Geometry check sheet. Reference: the model listing, model coordinates, mm. A direction names the side the tool comes from. Coordinates: 2 decimals unless noted, no trailing zeros. Write each loop counter-clockwise with the first axis right and the second up, starting at its lowest first coordinate (ties: lowest second). Pieces come first, ordered by that corner, then holes. Notation, with made-up numbers: M 65,12.25 L 72,12.25 A12 ccw 72,33.25 Z; hole C 30.5,-33.5 d3. An arc over 180 degrees is marked long. Put each result on its own line as item: value. Start each with the question number.
1) Cross-section at D-D on z = 43. Record the cut outline in (x, y), plus the area to 3 significant figures.
2) Scan lines: line 1 along Y through (x, z) = (0, 54); line 2 along X through (y, z) = (-25, 57); line 3 along X through (y, z) = (-41.5, 31). Record each from-to range of solid material in increasing order.
3) Set-up check for faces 5 (the flat face through (-5, 48.368, 75)), 6 (the cylindrical face through (-65.992, -68.182, 15.027)): record each of +Z, -Z, +X, -X, +Y, -Y from which the full face is reachable in a straight line by a thin tool's end or side.
4) Cross-section at A-A on x = 0. Record the cut outline in (y, z), plus the area to 3 significant figures.
5) Gauge pin test, flat ends, axial feed: pin 1 (10 mm diameter, centred on x = -87.5, y = -66, fed in from -Z); pin 2 (10 mm diameter, centred on y = -50, z = 106, fed in from -X). Record the tip position at first contact, or that the pin passes through.
6) Cross-section at B-B on y = 8. Record the cut outline in (x, z).
7) Mould release check, pull along X, two halves, no side actions. Record for faces 1 (the flat face through (-101, -69, 30.48)), 2 (the flat face through (-101, -58.402, 15)), 3 (the flat face through (-155.258, -29, 38)), 4 (the flat face through (149.542, -29, 75)): released by +X, released by -X, zero draft, split by the parting line, or undercut.
8) Cross-section at C-C on z = 25.5. Record the cut outline in (x, y), plus the area to 3 significant figures.
from build123d import *

# Parameters (mm, degrees)
F0_W     = 304.8
F0_H     = 152.4
F1_DEPTH = 152.4
F9_R     = 30.48
F5_DEPTH = 152.401
F6_SIZE  = 76.2
F8_DEPTH = 30.48


# Not quite as in the source:
# - the program builds the solid bodies; features that only make, move or delete a surface that nothing else refers to are left out


with BuildPart() as f1:
    # F0 (on Top) → F1 (new body)
    with BuildSketch(Plane.XY):
        with Locations((-2.8575006872, -27.8319329938)):
            Rectangle(F0_W, F0_H)
    extrude(amount=F1_DEPTH)

    # F9 (on face) → F5 (cut, through all)
    with BuildSketch(Plane.XY.offset(152.4)):
        with Locations((0, -15.3043069538)):
            Circle(F9_R)
    extrude(amount=-F5_DEPTH, mode=Mode.SUBTRACT)

    # F6
    f6_edges = [f1.edges().sort_by_distance(p)[0] for p in [
        (-155.257501, -27.831933, 152.4),
    ]]
    chamfer(f6_edges, length=F6_SIZE)

    # F7 (on face) → F8 (cut)
    with BuildSketch(Plane(origin=(0, 0, 0), x_dir=(1, 0, 0), z_dir=(0, 0, -1))):
        with BuildLine():
            ThreePointArc((-124.6516630054, 78.40236485), (-134.6516630054, 68.40236485), (-124.6516630054, 58.40236485))
            Line((-124.6516630054, 58.40236485), (-75.9895667434, 58.40236485))
            ThreePointArc((-75.9895667434, 58.40236485), (-65.9895667434, 68.40236485), (-75.9895667434, 78.40236485))
            Line((-75.9895667434, 78.40236485), (-124.6516630054, 78.40236485))
        make_face()
    extrude(amount=-F8_DEPTH, mode=Mode.SUBTRACT)


solid = f1.part
Answer key:
1. outline: M -155.26,-104.03 L 149.54,-104.03 L 149.54,48.37 L -155.26,48.37 Z; hole C 0,-15.3 d60.96
1. area: 43,500 mm²
2. line 1: y = -104.03 to -45.78, 15.18 to 48.37
2. line 2: x = -155.26 to -28.9, 28.9 to 149.54
2. line 3: x = -155.26 to -15.58, 15.58 to 149.54
3. face 5: +Z, -Z, +X, -X, +Y
3. face 6: -Z
4. outline: M -104.03,0 L -45.78,0 L -45.78,152.4 L -104.03,152.4 Z; M 15.18,0 L 48.37,0 L 48.37,152.4 L 15.18,152.4 Z
4. area: 13,900 mm²
5. pin 1: stops at z = 30.48
5. pin 2: stops at x = -130.46
6. outline: M -155.26,0 L -19.65,0 L -19.65,152.4 L -79.06,152.4 L -155.26,76.2 Z; M 19.65,0 L 149.54,0 L 149.54,152.4 L 19.65,152.4 Z
7. face 1: undercut
7. face 2: undercut
7. face 3: released by -X
7. face 4: released by +X
8. outline: M -155.26,-104.03 L 149.54,-104.03 L 149.54,48.37 L -155.26,48.37 Z; hole M -124.65,-78.4 L -75.99,-78.4 A10 ccw -75.99,-58.4 L -124.65,-58.4 A10 ccw Z; hole C 0,-15.3 d60.96
8. area: 42,200 mm²
